CAD build for the part. Positions are in the model's coordinates, mm. Face numbers are marked on the shaded views. A direction names the side the tool comes from. Coordinates: 2 decimals unless noted, no trailing zeros. Order: outer loops, then holes, each group sorted by start corner. A loop starts at its lowest first (then second) coordinate and runs counter-clockwise, first axis right, second up. Notation, with made-up numbers: (24.25, -7.5) - (37.25, -7.5) arc R29 ccw to (37.25, 19.5) - close; hole circle Ø1 at (57, -28.5). An arc over 180 degrees is marked (long way). Use one line per item in the form item = value.
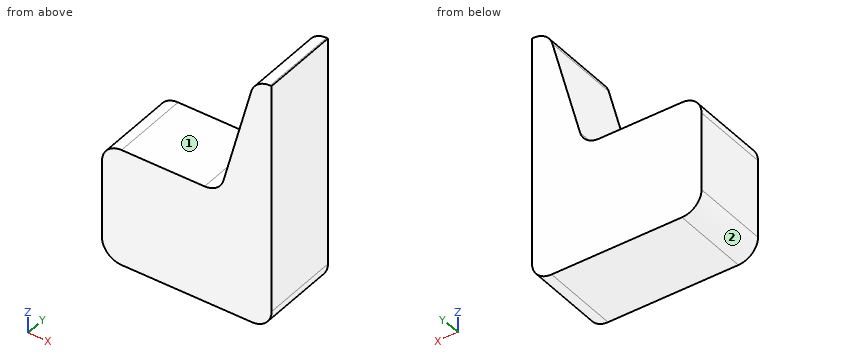
```python
from build123d import *

# Parameters (mm, degrees)
F2_DEPTH = 400
F3_R     = 100


# Not quite as in the source:
# - a feature of the source that left no trace in its solid (it failed there, or was rolled back) is left out
# - the program builds the solid bodies; features that only make, move or delete a surface that nothing else refers to are left out


with BuildPart() as f2:
    # F1 (on offset) → F2 (new body)
    with BuildSketch(Plane.XZ.offset(500)):
        Polygon((-781.1733315718, 197.8861267962), (-781.1733315718, -402.1138732038), (83.9892935576, -402.5302380195), (83.9892935576, 874.0342051986), (0, 874.0342051986), (-181.1733315718, 197.8861267962), align=None)
    extrude(amount=F2_DEPTH)

    # F3
    f3_edges = [f2.edges().sort_by_distance(p)[0] for p in [
        (-781.173332, -700, 197.886127),
        (0, -700, 874.034205),
        (-181.173332, -700, 197.886127),
        (-781.173332, -700, -402.113873),
        (83.989294, -700, -402.530238),
    ]]
    fillet(f3_edges, radius=F3_R)


solid = f2.part
```
Item 1: Cut at A-A, the plane y = -549.5. Write the cut outline in (x, z).
Derived:
outline = (-781.17, -302.16) arc R100 ccw to (-681.22, -402.16) - (-16.06, -402.48) arc R100 ccw to (83.99, -302.48) - (83.99, 874.03) - (76.73, 874.03) arc R100 ccw to (-19.86, 799.92) - (-161.31, 272) arc R100 cw to (-257.91, 197.89) - (-681.17, 197.89) arc R100 ccw to (-781.17, 97.89) - close
Item 2: Cut at C-C, the plane z = 536.5. Write the cut outline in (x, y).
Derived:
outline = (-90.44, -900) - (83.99, -900) - (83.99, -500) - (-90.44, -500) - close
Item 3: Drop a flat-ended pin along its axis: pin 1 (6 mm diameter, centred on x = -532.5, y = -852.5, fed in from +Z). Give the stop position or say it passes through.
Derived:
pin_1 = 197.89
Item 4: Drill centre lines: line 1 (Z direction, x = -500, y = -554.5); line 2 (Z direction, x = -453.5, y = -782.5); line 3 (X direction, y = -624, z = -336.5). Where is each one in solid material? Low to high. Write a range as [from, to].
Derived:
line_1 = [-402.25, 197.89]
line_2 = [-402.27, 197.89]
line_3 = [-775.09, 78.03]
Item 5: 3-axis set-ups, long thin cutter, end or side, ignore diameter. For the marked faces 1 and 2: which of +Z, -Z, +X, -X, +Y, -Y reach the whole face in a straight line?
Derived:
face_1 = +Z, -X, +Y, -Y
face_2 = -Z, -X, +Y, -Y
Item 6: Cut at B-B, the plane x = -479. Write the cut outline in (y, z).
Derived:
outline = (-900, -402.26) - (-500, -402.26) - (-500, 197.89) - (-900, 197.89) - close
